For this review, take the finished solid that the model builds, in its own axes (mm). Round coordinates to 2 decimals unless told otherwise and drop trailing zeros. Loops run counter-clockwise (first coordinate to the right, second up) from the corner with the lowest first, then second, coordinate; pieces in that order, holes last.
1) Take a section at D-D (y = 1.75). State the section outline as (x, z) points, then the cut area to 3 significant figures.
2) Mouldability with a two-part tool opening along X and no side actions: class faces 1 (the cylindrical face through (-2.34, 0.79, -0.37)), 2 (the cylindrical face through (-10, 1, 0)), 3 (the flat face through (-6, 1, 10)) as pulls with the +X half, pulls with the -X half, needs draft (parallel to the pull), parting line crosses it, or undercut.
3) Take a section at A-A (x = -4). State the section outline as (y, z) points.
4) Take a section at B-B (y = 0.3). State the section outline as (x, z) points.
5) Take a section at C-C (z = 0). State the section outline as (x, y) points.
6) Wall thickness on L1, parallel to Z at x = -4, y = 0.4; L2, parallel to X at y = 0.6, z = 0; L3, parallel to Z at x = -5, y = 1.5: over which ranges is each line inside the solid? List them lowest first.
```python
from build123d import *

# Parameters (mm, degrees)
BOSS_EXTRU_1_DEPTH = 3
CONG_1_R           = 1


with BuildPart() as part:
    # Esquisse1 → Boss.-Extru.1 (new body)
    with BuildSketch(Plane(origin=(0, 0, 0), x_dir=(1, 0, 0), z_dir=(0, 1, 0))):
        with BuildLine():
            Line((0, 10), (0, -10))
            Line((0, -10), (-12.679491924, -10))
            ThreePointArc((-12.679491924, -10), (-10, 0), (-12.679491924, 10))
            Line((-12.679491924, 10), (0, 10))
        make_face()
    extrude(amount=BOSS_EXTRU_1_DEPTH)

    # Esquisse3 → Fraisage pour vis à tête fraisée M31 (revolve, cut)
    with BuildSketch(Plane(origin=(-4, 3, 0), x_dir=(0, 0, 1), z_dir=(1, 0, 0))):
        Polygon((0, 0), (0, 3), (1.7, 3), (1.7, 1.45), (3.15, 0), align=None)
    revolve(axis=Axis((-4, 9.35, 0), (0, -1, 0)), mode=Mode.SUBTRACT)

    # Congé1
    # the kernel refuses this fillet: 1 mm, written as the material it takes off along each edge
    with BuildSketch(Plane(origin=(0, 3, -12.5), x_dir=(0, -1, 0), z_dir=(0, 0, 1))) as cong_1_piece_1:
        with BuildLine():
            CenterArc((CONG_1_R, -CONG_1_R), CONG_1_R, 90, 90)
            Line((0, -CONG_1_R), (0, 0))
            Line((0, 0), (CONG_1_R, 0))
        make_face()
    extrude(amount=25, mode=Mode.SUBTRACT)


solid = part.part
```
Response:
1. outline: (-12.68, -10) - (0, -10) - (0, 10) - (-12.68, 10) arc R20 cw to start; hole circle Ø3.8 at (-4, 0)
1. area: 206 mm2
2. face 1: undercut
2. face 2: pulls with the -X half
2. face 3: needs draft
3. outline: (0, -10) - (3, -10) - (3, -3.15) - (1.55, -1.7) - (0, -1.7) - close; (0, 1.7) - (1.55, 1.7) - (3, 3.15) - (3, 10) - (0, 10) - close
4. outline: (-12.68, -10) - (0, -10) - (0, 10) - (-12.68, 10) arc R20 cw to start; hole circle Ø3.4 at (-4, 0)
5. outline: (-10, 0) - (-5.7, 0) - (-5.7, 1.55) - (-7.15, 3) - (-10, 3) - close; (-2.3, 0) - (0, 0) - (0, 2) arc R1 ccw to (-0.86, 2.99) - (-2.3, 1.55) - close
6. L1: z = -10 to -1.7, 1.7 to 10
6. L2: x = -10 to -5.7, -2.3 to 0
6. L3: z = -10 to -1.37, 1.37 to 10
